Autodesk Fusion 360 part; units mm, degrees
sketch "スケッチ1" plane through (0, 0, 0) normal (0, 0, 1) x (1, 0, 0)
  line L0 (298, 149.5) -> (284, 149.5)
  line L1 (284, -149.5) -> (298, -149.5)
  line L2 (0, 149.5) -> (0, -149.5)
  line L3 (14, 17.5) -> (14, 149.5)
  line L4 (284, 149.5) -> (284, 17.5)
  line L5 (284, -17.5) -> (284, -149.5)
  line L6 (14, -149.5) -> (14, -17.5)
  line L7 (0, -149.5) -> (14, -149.5)
  line L8 (271, 4.5) -> (27, 4.5)
  line L9 (27, -4.5) -> (271, -4.5)
  line L10 (14, 149.5) -> (0, 149.5)
  line L11 (298, -149.5) -> (298, 149.5)
  arc A0 (27, -4.5) -> (14, -17.5) centre (27, -17.5) ccw
  arc A1 (14, 17.5) -> (27, 4.5) centre (27, 17.5) ccw
  arc A2 (271, 4.5) -> (284, 17.5) centre (271, 17.5) ccw
  arc A3 (284, -17.5) -> (271, -4.5) centre (271, -17.5) ccw
extrude "押し出し1" add sketch "スケッチ1" along normal blind 100
Work out the finished part from the listing and answer in its coordinate system (mm). A direction names the side the tool comes from. Round coordinates to 2 decimals unless told otherwise and drop trailing zeros. Loops run counter-clockwise (first coordinate to the right, second up) from the corner with the lowest first, then second, coordinate; pieces in that order, holes last. Notation, with made-up numbers: (63.5, 73.5) - (75.5, 73.5) arc R33 cw to (75.5, 109.5) - close; hole circle Ø9 at (30, 48.25). An arc over 180 degrees is marked (long way). Use one line per item in the form item = value. Start each with the question number.
(1) Find section D-D on y = 11. Determine the outline of the cut face in (x, z), and give its area (3 significant figures).
(2) Consider line 1 (X direction, y = -23.5, z = 46); line 2 (Y direction, x = 47, z = 26.5); line 3 (X direction, y = 15, z = 57.5). Determine where each line is inside the solid, lowest interval first.
(3) Find section C-C on x = 100. Determine the outline of the cut face in (y, z).
(4) Find section B-B on z = 42. Determine the outline of the cut face in (x, y), and give its area (3 significant figures).
(5) Flat-ended cylindrical pins translate along their axes: P1, Ø1, axis at x = 237.5, z = 58.5, coming from the -Y side; P2, Ø3, axis at x = 66, y = -7.5, coming from the +Z side. Find the tip coordinate at first contact, or state that the pin passes through.
(6) Determine the mould class of faces 1 (the face through (7, -149.5, 49)), 2 (the face through (298, -2, 49)), 3 (the face through (147, -4.5, 49)) for opening direction X: +X half, -X half, draft (parallel to the pull), parting line (faces both ways), or undercut.
(7) Which of the six approach directions +Z, -Z, +X, -X, +Y, -Y give full straight-line access (tool end or side, diameter ignored) to faces 4 (the face through (17.909, 8.207, 49.3)), 5 (the face through (17.707, -8.409, 49.3)), 6 (the face through (148, 1, 0))?
(8) Find section A-A on y = -79. Determine the outline of the cut face in (x, z), and give its area (3 significant figures).
Answer list:
q1.outline = (0, 0) - (15.74, 0) - (15.74, 100) - (0, 100) - close; (282.26, 0) - (298, 0) - (298, 100) - (282.26, 100) - close
q1.area = 3,150 mm^2
q2.line_1 = 0 to 14, 284 to 298
q2.line_2 = -4.5 to 4.5
q2.line_3 = 0 to 14.24, 283.76 to 298
q3.outline = (-4.5, 0) - (4.5, 0) - (4.5, 100) - (-4.5, 100) - close
q4.outline = (0, -149.5) - (14, -149.5) - (14, -17.5) arc R13 cw to (27, -4.5) - (271, -4.5) arc R13 cw to (284, -17.5) - (284, -149.5) - (298, -149.5) - (298, 149.5) - (284, 149.5) - (284, 17.5) arc R13 cw to (271, 4.5) - (27, 4.5) arc R13 cw to (14, 17.5) - (14, 149.5) - (0, 149.5) - close
q4.area = 10,900 mm^2
q5.P1 = -4.5
q5.P2 = through
q6.face_1 = draft
q6.face_2 = +X half
q6.face_3 = undercut
q7.face_4 = +Z, -Z, +Y
q7.face_5 = +Z, -Z, -Y
q7.face_6 = -Z, +X, -X, +Y, -Y
q8.outline = (0, 0) - (14, 0) - (14, 100) - (0, 100) - close; (284, 0) - (298, 0) - (298, 100) - (284, 100) - close
q8.area = 2,800 mm^2
